```python
from build123d import *

# Parameters (mm, degrees)
F0_R     = 12.7
F1_DEPTH = 4.7752
F2_R     = 2.38759
F3_R     = 4.7625
F4_DEPTH = 3.9751
F5_R     = 2.3876
F6_DEPTH = 17.4752


# Not quite as in the source:
# - a fillet or chamfer is up to 0.001 mm smaller than in the source, because OpenCascade refuses the exact size


with BuildPart() as f1:
    # F0 (on Front) → F1 (new body)
    with BuildSketch(Plane.XZ):
        Circle(F0_R)
    extrude(amount=F1_DEPTH)

    # F2 (radius 2.3876 in the source; OpenCascade refuses exactly that, so slightly less here)
    f2_edges = [f1.edges().sort_by_distance(p)[0] for p in [
        (-12.7, 0, 0),
        (-12.7, -4.7752, 0),
    ]]
    fillet(f2_edges, radius=F2_R)

    # F3 (on face) → F4 (join, symmetric)
    with BuildSketch(Plane.XZ.offset(4.7752)):
        Circle(F3_R)
    extrude(amount=F4_DEPTH, both=True)

    # F5 (on face) → F6 (join)
    with BuildSketch(Plane.XZ.offset(8.7503)):
        Circle(F5_R)
    extrude(amount=F6_DEPTH)


solid = f1.part
```
Check sheet for the modelled part. Datum: model origin and axes. Units: mm. A direction names the side the tool comes from. Give positions to 0.01 mm unless a question says otherwise; leave off trailing zeros. Order: outer loops, then holes, each group sorted by start corner. A loop starts at its lowest first (then second) coordinate and runs counter-clockwise, first axis right, second up. Notation, with made-up numbers: (-5.5, 74) -> (1.5, 74) arc R22 cw to (1.5, 81) -> close; hole circle Ø8 at (87.25, 12). An arc over 180 degrees is marked (long way). Return JSON: item names as keys, results as strings.
1. Cross-section at C-C, the plane y = -14. Record the cut outline in (x, z), plus the area to 3 significant figures.
From the geometry:
{"outline": "circle Ø4.78 at (0, 0)", "area": "17.9 mm^2"}
2. Go/stop test with flat-tipped pins: P1, Ø8, axis at y = -12, z = -1.5, coming from the +X side; P2, Ø12, axis at x = 3.5, y = -23, coming from the +Z side; P3, Ø10, axis at y = -8, z = -4.5, coming from the -X side. Record where each tip stops, or that it passes through.
From the geometry:
{"P1": "x = 4.76", "P2": "z = 2.39", "P3": "x = -12.21"}
3. Material ranges on probe 1 along Y at (x, z) = (-6, 0.5); probe 2 along Y at (x, z) = (3, -2.5); probe 3 along X at (y, z) = (-21, -1.5), recorded low to high. Write a range as [from, to].
From the geometry:
{"probe 1": "[-4.78, 0]", "probe 2": "[-8.75, 0]", "probe 3": "[-1.86, 1.86]"}
4. Cross-section at D-D, the plane y = -2.75. Record the cut outline in (x, z), plus the area to 3 significant figures.
From the geometry:
{"outline": "circle Ø25.34 at (0, 0)", "area": "505 mm^2"}
5. Set-up check for faces 1 (the flat face through (2, -8.75, -2)), 2 (the flat face through (0, 0, 0)): record each of +Z, -Z, +X, -X, +Y, -Y from which the full face is reachable in a straight line by a thin tool's end or side.
From the geometry:
{"face 1": "-Y", "face 2": "+Z, -Z, +X, -X, +Y"}
